```python
from build123d import *

# Parameters (mm, degrees)
BOSS_EXTRU_1_DEPTH       = 44
ESQUISSE2_R              = 7
ENL_V_MAT_EXTRU_1_DEPTH  = 44
ENL_V_MAT_EXTRU_2_DEPTH  = 19
ESQUISSE4_R              = 5.5
ENL_V_MAT_EXTRU_3_DEPTH  = 50
ENL_V_START              = -19
ENL_V_MAT_EXTRU_5_DEPTH  = 19
ENL_V_START_2            = -32
ENL_V_MAT_EXTRU_8_DEPTH  = 32
BOSS_EXTRU_3_START       = -8
BOSS_EXTRU_3_DEPTH       = 8
ESQUISSE15_R             = 5.5
ENL_V_MAT_EXTRU_9_DEPTH  = 44
ENL_V_MAT_EXTRU_10_DEPTH = 7
ENL_V_MAT_EXTRU_11_DEPTH = 32


with BuildPart() as part:
    # Esquisse1 → Boss.-Extru.1 (new body)
    with BuildSketch(Plane.XY):
        with BuildLine():
            Line((69.055498862, 42.585779817), (98.055498862, 42.585779817))
            Line((98.055498862, 42.585779817), (103.055498862, 37.585779817))
            Line((103.055498862, 37.585779817), (103.055498862, 18.585779817))
            Line((103.055498862, 18.585779817), (74.055498862, -15.414220183))
            Line((74.055498862, -15.414220183), (68.352478915, -15.414220183))
            ThreePointArc((68.352478915, -15.414220183), (64.19229693, -9.118662105), (61.797161375, -1.962930743))
            ThreePointArc((61.797161375, -1.962930743), (60.309086392, 2.242265049), (56.055498862, 3.585779817))
            Line((56.055498862, 3.585779817), (24.055498862, 3.585779817))
            Line((24.055498862, 3.585779817), (17.055498862, 10.585779817))
            Line((17.055498862, 10.585779817), (17.055498862, 28.585779817))
            Line((17.055498862, 28.585779817), (24.055498862, 35.585779817))
            Line((24.055498862, 35.585779817), (31.055498862, 35.585779817))
            Line((31.055498862, 35.585779817), (52.765077496, 31.757795364))
            ThreePointArc((52.765077496, 31.757795364), (62.410764196, 34.914360395), (69.055498862, 42.585779817))
        make_face()
    extrude(amount=BOSS_EXTRU_1_DEPTH)

    # Esquisse2 → Enlèv. mat.-Extru.1 (cut)
    with BuildSketch(Plane.XY.offset(44)):
        with Locations((31.055498862, 17.585779817)):
            Circle(ESQUISSE2_R)
    extrude(amount=-ENL_V_MAT_EXTRU_1_DEPTH, mode=Mode.SUBTRACT)

    # Esquisse3 → Enlèv. mat.-Extru.2 (cut)
    with BuildSketch(Plane.XY.offset(44)):
        Polygon((17.055498862, 28.585779817), (17.055498862, 10.585779817), (24.055498862, 3.585779817), (51.055498862, 3.585779817), (51.055498862, 32.059240202), (31.055498862, 35.585779817), (24.055498862, 35.585779817), align=None)
    extrude(amount=-ENL_V_MAT_EXTRU_2_DEPTH, mode=Mode.SUBTRACT)

    # Esquisse4 → Enlèv. mat.-Extru.3 (cut)
    with BuildSketch(Plane.XY.offset(44)):
        with Locations((89.055498862, 28.585779817)):
            Circle(ESQUISSE4_R)
    extrude(amount=-ENL_V_MAT_EXTRU_3_DEPTH, mode=Mode.SUBTRACT)

    # Esquisse10 → Enlèv. mat.-Extru.5 (cut)
    with BuildSketch(Plane.XY.offset(44).offset(ENL_V_START)):
        with BuildLine():
            Line((56.055498862, 3.585779817), (90.261381215, 3.585779817))
            Line((90.261381215, 3.585779817), (74.055498862, -15.414220183))
            Line((74.055498862, -15.414220183), (68.352478915, -15.414220183))
            ThreePointArc((68.352478915, -15.414220183), (64.19229693, -9.118662105), (61.797161375, -1.962930743))
            ThreePointArc((61.797161375, -1.962930743), (60.047831429, 1.971925154), (56.055498862, 3.585779817))
        make_face()
    extrude(amount=ENL_V_MAT_EXTRU_5_DEPTH, mode=Mode.SUBTRACT)

    # Esquisse13 → Enlèv. mat.-Extru.8 (cut)
    with BuildSketch(Plane.XY.offset(44).offset(ENL_V_START_2)):
        with BuildLine():
            Line((69.055498862, 42.585779817), (98.055498862, 42.585779817))
            Line((98.055498862, 42.585779817), (103.055498862, 37.585779817))
            Line((103.055498862, 37.585779817), (103.055498862, 18.585779817))
            Line((103.055498862, 18.585779817), (92.820204745, 6.585779817))
            ThreePointArc((92.820204745, 6.585779817), (74.207332122, 17.1537679), (63.456424114, 35.661587231))
            ThreePointArc((63.456424114, 35.661587231), (66.667333439, 38.791037909), (69.055498862, 42.585779817))
        make_face()
    extrude(amount=ENL_V_MAT_EXTRU_8_DEPTH, mode=Mode.SUBTRACT)

    # Esquisse14 → Boss.-Extru.3 (add)
    with BuildSketch(Plane.XY.offset(44).offset(BOSS_EXTRU_3_START)):
        with BuildLine():
            Line((92.820204745, 6.585779817), (103.055498862, 18.585779817))
            Line((103.055498862, 18.585779817), (103.055498862, 37.585779817))
            Line((103.055498862, 37.585779817), (98.055498862, 42.585779817))
            Line((98.055498862, 42.585779817), (69.055498862, 42.585779817))
            ThreePointArc((69.055498862, 42.585779817), (66.667333439, 38.791037909), (63.456424114, 35.661587231))
            ThreePointArc((63.456424114, 35.661587231), (74.207332122, 17.1537679), (92.820204745, 6.585779817))
        make_face()
    extrude(amount=BOSS_EXTRU_3_DEPTH)

    # Esquisse15 → Enlèv. mat.-Extru.9 (cut)
    with BuildSketch(Plane.XY.offset(44)):
        with Locations((89.055498862, 28.585779817)):
            Circle(ESQUISSE15_R)
    extrude(amount=-ENL_V_MAT_EXTRU_9_DEPTH, mode=Mode.SUBTRACT)

    # Esquisse16 → Enlèv. mat.-Extru.10 (cut)
    with BuildSketch(Plane.XY.offset(44)):
        with BuildLine():
            Line((52.055498862, 30.738438438), (52.055498862, 5.694877453))
            Line((52.055498862, 5.694877453), (52.055498862, 4.585779817))
            Line((52.055498862, 4.585779817), (89.799975158, 4.585779817))
            Line((89.799975158, 4.585779817), (99.846475633, 16.364435546))
            Line((99.846475633, 16.364435546), (102.055498862, 18.954324849))
            Line((102.055498862, 18.954324849), (102.055498862, 19.210406558))
            Line((102.055498862, 19.210406558), (102.055498862, 37.171566254))
            Line((102.055498862, 37.171566254), (97.6412853, 41.585779817))
            Line((97.6412853, 41.585779817), (69.792651449, 41.585779817))
            Line((69.792651449, 41.585779817), (69.676351802, 41.585779817))
            ThreePointArc((69.676351802, 41.585779817), (62.377758595, 33.70622702), (52.055498862, 30.738438438))
        make_face()
    extrude(amount=-ENL_V_MAT_EXTRU_10_DEPTH, mode=Mode.SUBTRACT)

    # Esquisse17 → Enlèv. mat.-Extru.11 (cut)
    with BuildSketch(Plane.XY.offset(37)):
        with BuildLine():
            ThreePointArc((62.594221181, 33.84139262), (57.542094296, 31.552111629), (52.055498862, 30.738438438))
            Line((52.055498862, 30.738438438), (52.055498862, 4.585779817))
            Line((52.055498862, 4.585779817), (89.799975158, 4.585779817))
            Line((89.799975158, 4.585779817), (90.652916335, 5.585779817))
            ThreePointArc((90.652916335, 5.585779817), (72.962922789, 16.078451846), (62.594221181, 33.84139262))
        make_face()
    extrude(amount=-ENL_V_MAT_EXTRU_11_DEPTH, mode=Mode.SUBTRACT)


solid = part.part
```
Can you work these out from the model? Positions are in its coordinate system, mm. A direction names the side the tool comes from. Give positions to 0.01 mm unless a question says otherwise; leave off trailing zeros. Loops run counter-clockwise (first coordinate to the right, second up) from the corner with the lowest first, then second, coordinate; pieces in that order, holes last. Notation, with made-up numbers: M 56.5,-7.5 L 102.5,-7.5 A21 cw 102.5,21.5 Z; hole C 69.5,42.5 d7. An arc over 180 degrees is marked long. Use CSV: the item, a comma, the result in double quotes. Start each with the question number.
1. Imagine slicing it at B-B, the plane z = 30. Write out the boundary of the cut face in (x, y).
2. On a 3-axis mill with a long thin cutter (end or side, diameter ignored), from which of +Z, -Z, +X, -X, +Y, -Y can I reach the whole of each face in a straight line? I mean faces 1 (the face through (74, -4, 25)), 2 (the face through (102.055, 28, 41)), 3 (the face through (74.424, 16.941, 23.832)). Say none if no direction works.
3. Imagine slicing it at C-C, the plane z = 3. Write out the boundary of the cut face in (x, y).
4. Imagine slicing it at D-D, the plane y = 8.5. Write out the boundary of the cut face in (x, z).
5. For P1, Ø16, axis at x = 34, y = 18.5, coming from the +Z side; P2, Ø4, axis at x = 32.5, z = 22.5, coming from the -Y side; P3, Ø6.5, axis at x = 89.06, y = 28.59, coming from the +Z side; P4, Ø5.5, axis at x = 26.5, z = 12, coming from the +Y side, each with a flat end and sliding along its axis, tell me the tip position at first contact or that it passes through.
6. If I drill on L1, parallel to X at y = 23, z = 39; L2, parallel to Y at x = 31, z = 23.5; L3, parallel to Z at x = 76, y = 39, over which ranges is the centre line in solid material (lowest first)?
7. Imagine slicing it at A-A, the plane x = 27. Write out the boundary of the cut face in (y, z).
8. If we mould it in two halves opening along Y, with no side actions, what happens to faces 4 (the face through (63, 16, 5)), 5 (the face through (64.239, -9.214, 12.325)), 6 (the face through (100.59, 40.05, 39.94))? For each: released by +Y, released by -Y, zero draft, split by the parting line, or undercut.
Response values:
1,outline,"M 51.06,3.59 L 56.06,3.59 A5 cw 57.61,3.59 L 90.26,3.59 L 92.82,6.59 A41 cw 63.46,35.66 A19 cw 52.77,31.76 L 51.06,32.06 Z; hole M 52.06,4.59 L 89.8,4.59 L 90.65,5.59 A41 cw 62.59,33.84 A20 cw 52.06,30.74 Z"
2,face 1,"+Z, +X, -X, -Y"
2,face 2,"+Z"
2,face 3,"+X, +Y"
3,outline,"M 17.06,10.59 L 24.06,3.59 L 56.06,3.59 A5 cw 61.8,-1.96 A29 ccw 68.35,-15.41 L 74.06,-15.41 L 103.06,18.59 L 103.06,37.59 L 98.06,42.59 L 69.06,42.59 A19 cw 52.77,31.76 L 31.06,35.59 L 24.06,35.59 L 17.06,28.59 Z; hole C 31.06,17.59 d14; hole C 89.06,28.59 d11"
4,outline,"M 19.14,0 L 94.45,0 L 94.45,12 L 87.15,12 L 87.15,36 L 94.45,36 L 94.45,44 L 93.14,44 L 93.14,37 L 83.32,37 L 83.32,5 L 52.06,5 L 52.06,44 L 51.06,44 L 51.06,25 L 19.14,25 Z"
5,P1,"z = 25"
5,P2,"y = 3.59"
5,P3,"through"
5,P4,"y = 35.59"
6,L1,"51.06 to 52.06, 102.06 to 103.06"
6,L2,"3.59 to 10.59, 24.59 to 35.59"
6,L3,"0 to 12, 36 to 37"
7,outline,"M 3.59,0 L 11.88,0 L 11.88,25 L 3.59,25 Z; M 23.29,0 L 35.59,0 L 35.59,25 L 23.29,25 Z"
8,face 4,"undercut"
8,face 5,"released by -Y"
8,face 6,"released by +Y"
